For this review, take the finished solid that the model builds, in its own axes (mm). A direction names the side the tool comes from. Give positions to 0.01 mm unless a question says otherwise; leave off trailing zeros. Loops run counter-clockwise (first coordinate to the right, second up) from the corner with the lowest first, then second, coordinate; pieces in that order, holes last.
```python
from build123d import *

# Parameters (mm, degrees)
CROQUIS1_W              = 28.5
CROQUIS1_H              = 28.5
SALIENTE_EXTRUIR1_DEPTH = 1.5
SALIENTE_EXTRUIR2_DEPTH = 4
CROQUIS3_W              = 25
CROQUIS3_H              = 25
SALIENTE_EXTRUIR3_DEPTH = 4.1
CROQUIS4_W              = 4
CROQUIS4_H              = 6
SALIENTE_EXTRUIR4_DEPTH = 0.1
VACIADO2_START          = -3.1
VACIADO2_DEPTH          = 7.6
VACIADO2_2_DEPTH        = 3.6
VACIADO2_START_2        = 1
VACIADO2_3_OUTLINE_W    = 0.7
VACIADO2_3_OUTLINE_H    = 4
VACIADO2_3_DEPTH        = 3.5


# Read off the part's stored shape, not the designer's step: Vaciado2
with BuildPart() as part:
    # Croquis1 → Saliente-Extruir1 (new body)
    with BuildSketch(Plane.XY):
        Rectangle(CROQUIS1_W, CROQUIS1_H)
    extrude(amount=SALIENTE_EXTRUIR1_DEPTH)

    # Croquis2 → Saliente-Extruir2 (add)
    with BuildSketch(Plane.XY.offset(1.5)):
        Polygon((-12.1, 9.466756826), (-9.466756826, 12.1), (9.466756826, 12.1), (12.1, 9.466756826), (12.1, -9.466756826), (9.466756826, -12.1), (-9.466756826, -12.1), (-12.1, -9.466756826), align=None)
    extrude(amount=SALIENTE_EXTRUIR2_DEPTH)

    # Croquis3 → Saliente-Extruir3 (add)
    with BuildSketch(Plane(origin=(0, 0, 0), x_dir=(-1, 0, 0), z_dir=(0, 0, -1))):
        Rectangle(CROQUIS3_W, CROQUIS3_H)
    extrude(amount=SALIENTE_EXTRUIR3_DEPTH)

    # Croquis4 → Saliente-Extruir4 (add)
    with BuildSketch(Plane.ZY.offset(12.1)):
        with Locations((3.5, 0)):
            Rectangle(CROQUIS4_W, CROQUIS4_H)
    extrude(amount=SALIENTE_EXTRUIR4_DEPTH)

    # Vaciado2 outline → Vaciado2 (cut)
    with BuildSketch(Plane.XY.offset(VACIADO2_START)):
        Polygon((-11.1, 2), (-11.5, 2), (-11.5, -2), (-11.1, -2), (-11.1, -9.052543264), (-9.052543264, -11.1), (9.052543264, -11.1), (11.1, -9.052543264), (11.1, 9.052543264), (9.052543264, 11.1), (-9.052543264, 11.1), (-11.1, 9.052543264), align=None)
    extrude(amount=VACIADO2_DEPTH, mode=Mode.SUBTRACT)

    # Vaciado2 2 outline → Vaciado2 2 (cut)
    with BuildSketch(Plane.XY.offset(VACIADO2_START)):
        Polygon((-11.5, 11.5), (-11.5, 2), (-11.1, 2), (-11.1, 9.052543264), (-9.052543264, 11.1), (9.052543264, 11.1), (11.1, 9.052543264), (11.1, -9.052543264), (9.052543264, -11.1), (-9.052543264, -11.1), (-11.1, -9.052543264), (-11.1, -2), (-11.5, -2), (-11.5, -11.5), (11.5, -11.5), (11.5, 11.5), align=None)
    extrude(amount=VACIADO2_2_DEPTH, mode=Mode.SUBTRACT)

    # Vaciado2 3 outline → Vaciado2 3 (cut)
    with BuildSketch(Plane.XY.offset(VACIADO2_START_2)):
        with Locations((-11.85, 0)):
            Rectangle(VACIADO2_3_OUTLINE_W, VACIADO2_3_OUTLINE_H)
    extrude(amount=VACIADO2_3_DEPTH, mode=Mode.SUBTRACT)


solid = part.part
```
Item 1: Take a section at C-C on z = -1. Give the boundary of the cut face in (x, y), and give its area (3 significant figures).
Answer:
outline: (-12.5, -12.5) - (12.5, -12.5) - (12.5, 12.5) - (-12.5, 12.5) - close; hole (-11.5, -11.5) - (11.5, -11.5) - (11.5, 11.5) - (-11.5, 11.5) - close
area: 96.0 mm2
Item 2: The part is to be moulded in two halves that separate along Z. For faces 6 (the flat face through (11.1, 0, 2)), 7 (the flat face through (10.765, 10.802, 3.472)), 8 (the flat face through (-1, 0, 4.5)), say which applies: released by +Z, released by -Z, zero draft, split by the parting line, or undercut.
Answer:
face 6: undercut
face 7: zero draft
face 8: undercut
Item 3: Take a section at D-D on z = 4. Give the boundary of the cut face in (x, y), and give its area (3 significant figures).
Answer:
outline: (-12.2, -3) - (-12.1, -3) - (-12.1, -9.47) - (-9.47, -12.1) - (9.47, -12.1) - (12.1, -9.47) - (12.1, 9.47) - (9.47, 12.1) - (-9.47, 12.1) - (-12.1, 9.47) - (-12.1, 3) - (-12.2, 3) - (-12.2, 2) - (-11.1, 2) - (-11.1, 9.05) - (-9.05, 11.1) - (9.05, 11.1) - (11.1, 9.05) - (11.1, -9.05) - (9.05, -11.1) - (-9.05, -11.1) - (-11.1, -9.05) - (-11.1, -2) - (-12.2, -2) - close
area: 83.5 mm2
Item 4: Clearance check with flat-ended pins moving along their axes: pin 1 Ø2 at (y, z) = (-5.5, -1.5) entering from +X; pin 2 Ø0.5 at (x, z) = (-11.5, 3) entering from +Y; pin 3 Ø3 at (x, z) = (-4, 4) entering from +Y. State where each tip first meets the part, or that it passes through.
Answer:
pin 1: stops at x = 12.5
pin 2: stops at y = 10.32
pin 3: stops at y = 12.1
Item 5: Tool access review of faces 1 (the flat face through (-12.1, -6, 3)), 2 (the flat face through (12.5, 0, -2)), 3 (the flat face through (0, 11.5, -1)), 4 (the flat face through (0, -12.1, 3)), 5 (the flat face through (-10.802, 10.765, 3.472)): name each direction out of +Z, -Z, +X, -X, +Y, -Y from which nothing blocks a thin tool from reaching the whole face with its end or side.
Answer:
face 1: +Z, -X, -Y
face 2: -Z, +X, +Y, -Y
face 3: none
face 4: +Z, +X, -X, -Y
face 5: +Z, -X, +Y
Item 6: For L1, parallel to Z at x = -2, y = -0.5; L2, parallel to X at y = -2.5, z = -1.5; L3, parallel to Y at x = 9, z = 1.25, list the stretches that pass through material, from the lowest coordinate up.
Answer:
L1: z = -4.1 to -3.1, 4.5 to 5.5
L2: x = -12.5 to -11.5, 11.5 to 12.5
L3: y = -14.25 to -11.1, 11.1 to 14.25
Item 7: Take a section at A-A on y = -5.75. Give the boundary of the cut face in (x, z), and give its area (4 significant figures).
Answer:
outline: (-14.25, 0) - (-12.5, 0) - (-12.5, -4.1) - (12.5, -4.1) - (12.5, 0) - (14.25, 0) - (14.25, 1.5) - (12.1, 1.5) - (12.1, 5.5) - (-12.1, 5.5) - (-12.1, 1.5) - (-14.25, 1.5) - close; hole (-11.5, -3.1) - (11.5, -3.1) - (11.5, 0.5) - (11.1, 0.5) - (11.1, 4.5) - (-11.1, 4.5) - (-11.1, 0.5) - (-11.5, 0.5) - close
area: 70.45 mm2
